from build123d import *

# Parameters (mm, degrees)
EXTRUDE_1_DEPTH = 10


with BuildPart() as part:
    # Эскиз1 → Бобышка-Вытянуть1 (new, symmetric)
    with BuildSketch(Plane.XY):
        with BuildLine():
            Line((14.4, -1.65), (23.75, -1.65))
            ThreePointArc((23.75, -1.65), (24.209619408, -1.840380592), (24.4, -2.3))
            Line((24.4, -2.3), (24.4, -2.7))
            ThreePointArc((24.4, -2.7), (24.209619408, -3.159619408), (23.75, -3.35))
            Line((23.75, -3.35), (14.4, -3.35))
            Line((14.4, -3.35), (14.4, -3.25))
            Line((14.4, -3.25), (23.7, -3.25))
            ThreePointArc((23.7, -3.25), (24.124264069, -3.074264069), (24.3, -2.65))
            Line((24.3, -2.65), (24.3, -2.35))
            ThreePointArc((24.3, -2.35), (24.124264069, -1.925735931), (23.7, -1.75))
            Line((23.7, -1.75), (14.4, -1.75))
            Line((14.4, -1.75), (14.4, -1.65))
        make_face()
    extrude(amount=EXTRUDE_1_DEPTH, both=True)


solid = part.part
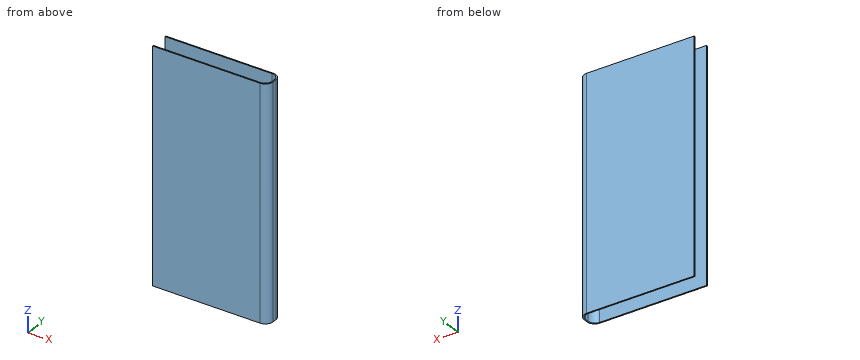
Verification items for the finished model (mm, model axes). Give positions to 0.01 mm unless a question says otherwise; leave off trailing zeros. Order: outer loops, then holes, each group sorted by start corner. A loop starts at its lowest first (then second) coordinate and runs counter-clockwise, first axis right, second up. Notation, with made-up numbers: M 30.25,28.5 L 70.25,28.5 A14 cw 70.25,44.5 Z; hole C -24.5,-7 d2. An arc over 180 degrees is marked long. Use one line per item in the form item = value. Start each with the question number.
Q1. Section check B-B (z = -2). Enter the section's corners in (x, y), then the cut area to 3 significant figures.
Q2. Section check A-A (x = 23.25). Enter the section's corners in (y, z), then the cut area to 3 significant figures.
Q3. Section check C-C (y = -3). Enter the section's corners in (x, z).
Q4. Scan lines: line 1 along X through (y, z) = (-3.1, -5.25); line 2 along X through (y, z) = (-3.15, -8.25). Record each from-to range of solid material in increasing order. Write a range as [from, to].
Evaluation:
q1.outline = M 14.4,-3.35 L 23.75,-3.35 A0.65 ccw 24.4,-2.7 L 24.4,-2.3 A0.65 ccw 23.75,-1.65 L 14.4,-1.65 L 14.4,-1.75 L 23.7,-1.75 A0.6 cw 24.3,-2.35 L 24.3,-2.65 A0.6 cw 23.7,-3.25 L 14.4,-3.25 Z
q1.area = 2.12 mm2
q2.outline = M -3.35,-10 L -3.25,-10 L -3.25,10 L -3.35,10 Z; M -1.75,-10 L -1.65,-10 L -1.65,10 L -1.75,10 Z
q2.area = 4.00 mm2
q3.outline = M 24.19,-10 L 24.33,-10 L 24.33,10 L 24.19,10 Z
q4.line_1 = [24.1, 24.26]
q4.line_2 = [24.03, 24.22]
